Geometry: final body of the model. Coordinates: model frame, mm. A direction names the side the tool comes from. Give positions to 0.01 mm unless a question says otherwise; leave off trailing zeros. Write each loop counter-clockwise with the first axis right and the second up, starting at its lowest first coordinate (ties: lowest second). Pieces come first, ordered by that corner, then holes. Notation, with made-up numbers: M 27.5,73.25 L 85.5,73.25 A25 ccw 85.5,100.25 Z; hole C 14,88 d1. An arc over 180 degrees is marked long. Use a Markdown table: item, result. Add a question column.
1) Line query: line 1 (Y direction, x = 19.5, z = 12); line 2 (X direction, y = 43.5, z = 8.75); line 3 (X direction, y = 17, z = 13). Output: solid intervals per line, ascending.
2) Section D-D on y = 41. Return the cut outline in (x, z), then the cut area to 3 significant figures.
3) Section C-C on x = 26. Return the cut outline in (y, z).
4) Section A-A on z = 7.7. Return the cut outline in (x, y).
5) Pin query (flat end, axial travel): pin 1 (1.5 mm diameter, centred on y = 17.5, z = 12.5, fed in from +X); pin 2 (6 mm diameter, centred on x = -16.5, z = 9, fed in from +Y); pin 3 (15 mm diameter, centred on x = 2.73, y = 36, fed in from -Z); pin 4 (7.5 mm diameter, centred on y = 30.5, z = 6.5, fed in from -X). Return the tip coordinate at first contact, or that it passes through.
6) Draft query along X for faces 1 (the cylindrical face through (2.403, 50.996, 7.592)), 2 (the cylindrical face through (0.691, 26.806, 7.808)), 3 (the flat face through (3, 0, 8)). Return one class per face: +X half, -X half, draft (parallel to the pull), parting line (faces both ways), or undercut.
7) Section B-B on z = 14.25. Return the cut outline in (x, y), then the cut area to 3 significant figures.
8) Set-up query: faces 4 (the cylindrical face through (-26.763, 7.888, 7.898)), 5 (the flat face through (-17, 16, 8)), 6 (the flat face through (22, 16, 8)). Return all of +Z, -Z, +X, -X, +Y, -Y with unobstructed straight access to the full face (end or side cutting, diameter ignored); none if empty.
```python
from build123d import *

# Parameters (mm, degrees)
SALIENTE_EXTRUIR1_DEPTH = 15.4
CROQUIS2_R              = 9.417866401
CORTAR_EXTRUIR1_DEPTH   = 16.4
CROQUIS3_R              = 4.5
CORTAR_EXTRUIR2_DEPTH   = 52


with BuildPart() as part:
    # Croquis1 → Saliente-Extruir1 (new body)
    with BuildSketch(Plane.XY):
        with BuildLine():
            Line((-30.267515924, 0), (-30.267515924, 15))
            ThreePointArc((-30.267515924, 15), (-29.974622705, 15.707106781), (-29.267515924, 16))
            Line((-29.267515924, 16), (-12.267515924, 16))
            Line((-12.267515924, 16), (-12.267515924, 36))
            ThreePointArc((-12.267515924, 36), (2.732484076, 51), (17.732484076, 36))
            Line((17.732484076, 36), (17.732484076, 16))
            Line((17.732484076, 16), (34.732484076, 16))
            ThreePointArc((34.732484076, 16), (35.439590858, 15.707106781), (35.732484076, 15))
            Line((35.732484076, 15), (35.732484076, 0))
            Line((35.732484076, 0), (-30.267515924, 0))
        make_face()
    extrude(amount=SALIENTE_EXTRUIR1_DEPTH)

    # Croquis2 → Cortar-Extruir1 (cut, through all)
    with BuildSketch(Plane.XY.offset(15.4)):
        with Locations((2.732484076, 36)):
            Circle(CROQUIS2_R)
    extrude(amount=-CORTAR_EXTRUIR1_DEPTH, mode=Mode.SUBTRACT)

    # Croquis3 → Cortar-Extruir2 (cut, through all)
    with BuildSketch(Plane.XZ):
        with Locations((-22.267515924, 7.7)):
            Circle(CROQUIS3_R)
        with Locations((27.732484076, 7.7)):
            Circle(CROQUIS3_R)
    extrude(amount=-CORTAR_EXTRUIR2_DEPTH, mode=Mode.SUBTRACT)


solid = part.part
```
Found:
| question | item | result |
|---|---|---|
| 1 | line 1 | 0 to 16 |
| 1 | line 2 | -10.26 to -2.96, 8.43 to 15.72 |
| 1 | line 3 | -12.27 to 17.73 |
| 2 | outline | M -11.41,0 L -5.25,0 L -5.25,15.4 L -11.41,15.4 Z; M 10.71,0 L 16.87,0 L 16.87,15.4 L 10.71,15.4 Z |
| 2 | area | 190 mm² |
| 3 | outline | M 0,0 L 16,0 L 16,3.55 L 0,3.55 Z; M 0,11.85 L 16,11.85 L 16,15.4 L 0,15.4 Z |
| 4 | outline | M -30.27,0 L -26.77,0 L -26.77,16 L -29.27,16 A1 ccw -30.27,15 Z; M -17.77,0 L 23.23,0 L 23.23,16 L 17.73,16 L 17.73,36 A15 ccw -12.27,36 L -12.27,16 L -17.77,16 Z; M 32.23,0 L 35.73,0 L 35.73,15 A1 ccw 34.73,16 L 32.23,16 Z; hole C 2.73,36 d18.84 |
| 5 | pin 1 | x = 17.73 |
| 5 | pin 2 | y = 16 |
| 5 | pin 3 | through |
| 5 | pin 4 | x = -12.27 |
| 6 | face 1 | parting line |
| 6 | face 2 | undercut |
| 6 | face 3 | draft |
| 7 | outline | M -30.27,0 L 35.73,0 L 35.73,15 A1 ccw 34.73,16 L 17.73,16 L 17.73,36 A15 ccw -12.27,36 L -12.27,16 L -29.27,16 A1 ccw -30.27,15 Z; hole C 2.73,36 d18.84 |
| 7 | area | 1,730 mm² |
| 8 | face 4 | +Y, -Y |
| 8 | face 5 | +Z, -Z, -X, +Y |
| 8 | face 6 | +Z, -Z, +X, +Y |
